Build history of the part. All positions in model axes, mm. Face numbers are marked on the shaded views. A direction names the side the tool comes from. Give positions to 0.01 mm unless a question says otherwise; leave off trailing zeros. Loops run counter-clockwise (first coordinate to the right, second up) from the corner with the lowest first, then second, coordinate; pieces in that order, holes last. Notation, with made-up numbers: M 29,66 L 67,66 A28 ccw 67,92 Z; hole C -28.75,54.25 d7. An arc over 180 degrees is marked long. Put each result on its own line as item: value.
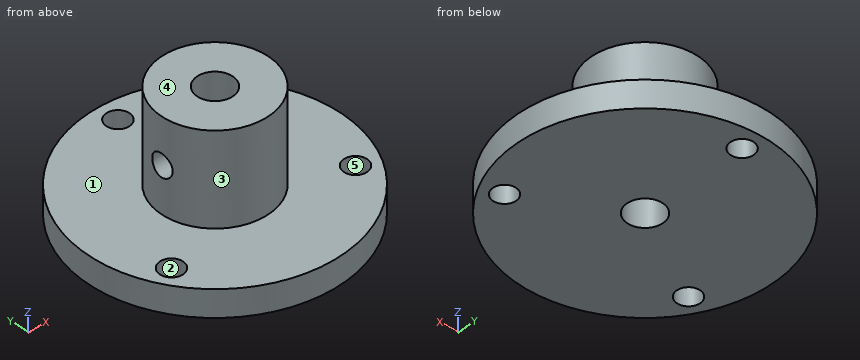
```python
from build123d import *

# Parameters (mm, degrees)
SKETCH2_R           = 28.4
BOSS_EXTRUDE1_DEPTH = 6
SKETCH3_R           = 12
BOSS_EXTRUDE2_DEPTH = 20.4
SKETCH4_R           = 4
CUT_EXTRUDE1_DEPTH  = 49.063291606
SKETCH5_R           = 2.6
CUT_EXTRUDE2_DEPTH  = 49.063291606
CIRPATTERN2_COUNT   = 3
SKETCH6_R           = 2.5
CUT_EXTRUDE3_DEPTH  = 49.063291606


with BuildPart() as part:
    # Sketch2 → Boss-Extrude1 (new body)
    with BuildSketch(Plane.XY):
        Circle(SKETCH2_R)
    extrude(amount=BOSS_EXTRUDE1_DEPTH)

    # Sketch3 → Boss-Extrude2 (add)
    with BuildSketch(Plane.XY.offset(6)):
        Circle(SKETCH3_R)
    extrude(amount=BOSS_EXTRUDE2_DEPTH)

    # Sketch4 → Cut-Extrude1 (cut, through all)
    with BuildSketch(Plane.XY.offset(26.4)):
        Circle(SKETCH4_R)
    extrude(amount=-CUT_EXTRUDE1_DEPTH, mode=Mode.SUBTRACT)

    # Sketch5 → Cut-Extrude2 (cut, through all)
    with BuildSketch(Plane(origin=(0, 0, 0), x_dir=(-1, 0, 0), z_dir=(0, 0, -1))):
        with Locations((0, 23.75)):
            Circle(SKETCH5_R)
    cut_extrude2 = extrude(amount=-CUT_EXTRUDE2_DEPTH, mode=Mode.SUBTRACT)

    # CirPattern2: Cut-Extrude2 ×3 about axis
    cirpattern2_axis = Axis((0, 0, 0), (0, 0, 1))
    for i in range(1, CIRPATTERN2_COUNT):
        add(cut_extrude2.rotate(cirpattern2_axis, i * 360 / CIRPATTERN2_COUNT), mode=Mode.SUBTRACT)

    # Sketch6 → Cut-Extrude3 (cut, through all)
    with BuildSketch(Plane(origin=(0, 0, 0), x_dir=(0, 0, -1), z_dir=(1, 0, 0))):
        with Locations((-16.2, 0)):
            Circle(SKETCH6_R)
    extrude(amount=-CUT_EXTRUDE3_DEPTH, mode=Mode.SUBTRACT)


solid = part.part
```
Q1. Drop flat-ended pins along their axis: pin 1 Ø7 at (x, y) = (0, 0) entering from -Z; pin 2 Ø4 at (x, z) = (-6.5, 11.5) entering from +Y; pin 3 Ø6 at (x, y) = (-17, -8) entering from +Z; pin 4 Ø1 at (x, z) = (-5.5, 9.5) entering from -Y. Give the stop position or say it passes through.
Here are the results:
pin 1: through
pin 2: y = 11.12
pin 3: z = 6
pin 4: y = -10.91
Q2. Probe line 1 (Y direction, x = 0, z = 4); line 2 (Y direction, x = 0, z = 25.25); line 3 (Z direction, x = -9.5, y = 21.5). List the from-to ranges inside material, lowest first. Write a range as from..to.
Here are the results:
line 1: -28.4..-4, 4..21.15, 26.35..28.4
line 2: -12..-4, 4..12
line 3: 0..6
Q3. Mould opens along X. For the marked faces 3, 4 and 5 say: pulls with the +X half, pulls with the -X half, needs draft (parallel to the pull), parting line crosses it, or undercut.
Here are the results:
face 3: parting line crosses it
face 4: needs draft
face 5: undercut
Q4. Slice it at D-D (z = 21.75). List the corners of the cut face in (x, y).
Here are the results:
outline: C 0,0 d24; hole C 0,0 d8
Q5. Slice it at A-A (y = 23.75). List the corners of the cut face in (x, z).
Here are the results:
outline: M -15.57,0 L -2.6,0 L -2.6,6 L -15.57,6 Z; M 2.6,0 L 15.57,0 L 15.57,6 L 2.6,6 Z
Q6. Slice it at C-C (x = 19.5). List the corners of the cut face in (y, z).
Here are the results:
outline: M -20.65,0 L -14.25,0 L -14.25,6 L -20.65,6 Z; M -9.5,0 L 20.65,0 L 20.65,6 L -9.5,6 Z
Q7. Slice it at B-B (y = 0). List the corners of the cut face in (x, z).
Here are the results:
outline: M -28.4,0 L -4,0 L -4,13.7 L -12,13.7 L -12,6 L -28.4,6 Z; M -12,18.7 L -4,18.7 L -4,26.4 L -12,26.4 Z; M 4,0 L 28.4,0 L 28.4,6 L 12,6 L 12,26.4 L 4,26.4 Z
Q8. Tool access for the marked faces 1 and 2: list every direction of +Z, -Z, +X, -X, +Y, -Y with a clear straight run to the whole face (end or side of a thin tool).
Here are the results:
face 1: +Z
face 2: +Z, -Z
